```python
from build123d import *

# Parameters (mm, degrees)
CROQUIS1_W              = 70
CROQUIS1_H              = 100
SALIENTE_EXTRUIR1_DEPTH = 10
CROQUIS2_W              = 51
CROQUIS2_H              = 90.5
CORTAR_EXTRUIR1_DEPTH   = 10
REDONDEO1_R             = 5


with BuildPart() as part:
    # Croquis1 → Saliente-Extruir1 (new body)
    with BuildSketch(Plane(origin=(0, 0, 0), x_dir=(1, 0, 0), z_dir=(0, 1, 0))):
        with Locations((35, -50)):
            Rectangle(CROQUIS1_W, CROQUIS1_H)
    extrude(amount=SALIENTE_EXTRUIR1_DEPTH)

    # Croquis2 → Cortar-Extruir1 (cut)
    with BuildSketch(Plane(origin=(0, 10, 0), x_dir=(1, 0, 0), z_dir=(0, 1, 0))):
        with Locations((35, -54.75)):
            Rectangle(CROQUIS2_W, CROQUIS2_H)
    extrude(amount=-CORTAR_EXTRUIR1_DEPTH, mode=Mode.SUBTRACT)

    # Redondeo1
    # the kernel refuses this fillet: 5 mm, written as the material it takes off along each edge
    with BuildSketch(Plane(origin=(9.5, 22.5, 100), x_dir=(-1, 0, 0), z_dir=(0, -1, 0)), Plane(origin=(70, -12.5, 100), x_dir=(0, 0, -1), z_dir=(0, 1, 0)), Plane(origin=(70, -12.5, 0), x_dir=(-1, 0, 0), z_dir=(0, 1, 0))) as redondeo1_piece_1:
        with BuildLine():
            CenterArc((REDONDEO1_R, REDONDEO1_R), REDONDEO1_R, 180, 90)
            Line((0, REDONDEO1_R), (0, 0))
            Line((0, 0), (REDONDEO1_R, 0))
        make_face()
    extrude(amount=35, mode=Mode.SUBTRACT)
    with BuildSketch(Plane(origin=(60.5, 22.5, 100), x_dir=(1, 0, 0), z_dir=(0, -1, 0)), Plane(origin=(0, -12.5, 0), x_dir=(1, 0, 0), z_dir=(0, 1, 0)), Plane(origin=(0, -12.5, 100), x_dir=(0, 0, -1), z_dir=(0, 1, 0))) as redondeo1_piece_2:
        with BuildLine():
            CenterArc((REDONDEO1_R, -REDONDEO1_R), REDONDEO1_R, 90, 90)
            Line((0, -REDONDEO1_R), (0, 0))
            Line((0, 0), (REDONDEO1_R, 0))
        make_face()
    extrude(amount=35, mode=Mode.SUBTRACT)


solid = part.part
```
Read the model definition and answer for the solid it produces. Units are mm, in the model's axes. A direction names the side the tool comes from. Give positions to 0.01 mm unless a question says otherwise; leave off trailing zeros. Write each loop counter-clockwise with the first axis right and the second up, starting at its lowest first coordinate (ties: lowest second). Pieces come first, ordered by that corner, then holes. Notation, with made-up numbers: M 64,41.5 L 85,41.5 A28 ccw 85,63.5 Z; hole C 49.25,-28 d4. An arc over 180 degrees is marked long. Put each result on its own line as item: value. Start each with the question number.
1. The part is cut by section A-A, the plane y = 6. Give the vertices of the cut face in (x, z).
2. Which of the six approach directions +Z, -Z, +X, -X, +Y, -Y give full straight-line access (tool end or side, diameter ignored) to faces 1 (the flat face through (60.5, 5, 53)), 2 (the flat face through (0, 5, 51))?
3. The part is cut by section C-C, the plane x = 56.5. Give the vertices of the cut face in (y, z).
4. This flat-tipped pin is pushed along its axis until it touches: pin 1 Ø5 at (x, y) = (42.5, 4.5) entering from +Z. Where does it stop, or does it pass through?
5. Consider line 1 along X through (y, z) = (9, 81); line 2 along Z through (x, y) = (50, 4.5); line 3 along Z through (x, y) = (3.5, 5). Determine where each line is inside the solid, lowest interval first.
6. For a pull along X with two mould halves and no side action, classify faces 3 (the flat face through (70, 5, 51)), 4 (the cylindrical face through (8.159, 5.07, 98.407)), 5 (the flat face through (61, 0, 39)) as released by +X, released by -X, zero draft, split by the parting line, or undercut.
7. The part is cut by section B-B, the plane z = 64. Give the vertices of the cut face in (x, y), and give its area (3 significant figures).
Final values:
1. outline: M 0,5 A5 ccw 5,0 L 65,0 A5 ccw 70,5 L 70,95 A5 ccw 65.25,99.99 A5 ccw 60.5,95 L 60.5,9.5 L 9.5,9.5 L 9.5,95 A5 ccw 4.75,99.99 A5 ccw 0,95 Z
2. face 1: +Z, +Y, -Y
2. face 2: +Z, -Z, -X, +Y, -Y
3. outline: M 0,0 L 10,0 L 10,9.5 L 0,9.5 Z
4. pin 1: stops at z = 9.5
5. line 1: x = 0 to 9.5, 60.5 to 70
5. line 2: z = 0 to 9.5
5. line 3: z = 0.23 to 99.77
6. face 3: released by +X
6. face 4: undercut
6. face 5: zero draft
7. outline: M 0,0 L 9.5,0 L 9.5,10 L 0,10 Z; M 60.5,0 L 70,0 L 70,10 L 60.5,10 Z
7. area: 190 mm²
